Could you check a few things on this drawing? It's one solid part, dimensions in mm from its lowest x, y, z. Give positions to 0.01 mm unless a question says otherwise; leave off trailing zeros. Loops run counter-clockwise (first coordinate to the right, second up) from the corner with the lowest first, then second, coordinate; pieces in that order, holes last. Notation, with made-up numbers: M 85,49 L 134,49 A13 ccw 134,63 Z; hole C 1.5,73.25 d5. An arc over 180 degrees is marked long. Answer as CSV lines item,"result". Start each with the question number.
Item 1: I want a section at B-B on x = 15.25. List the corners of the cut face in (y, z) for me.
Item 2: I want a section at D-D on x = 4. List the corners of the cut face in (y, z) for me, plus the area to 3 significant figures.
Item 3: I want a section at C-C on z = 11.9. List the corners of the cut face in (x, y) for me.
Item 4: If I drill on line 1 along X through (y, z) = (4.55, 42.5); line 2 along Z through (x, y) = (11, 1.25); line 3 along X through (y, z) = (0.45, 11.9), over which ranges is the centre line in solid material (lowest first)? Write a range as from..to.
Item 5: Will these pins go through, and if not, where does the flat tip stop? P1, Ø12, axis at x = 7.5, z = 14, coming from the +Y side; P2, Ø6, axis at x = 15, z = 5, coming from the -Y side; P3, Ø5, axis at x = 18, z = 38.5, coming from the -Y side.
Item 6: If we mould it in two halves opening along Z, with no side actions, what happens to the marked faces 1, 2 and 3? For each: released by +Z, released by -Z, zero draft, split by the parting line, or undercut.
Item 7: I want a section at A-A on y = 3.45. List the corners of the cut face in (x, z) for me.
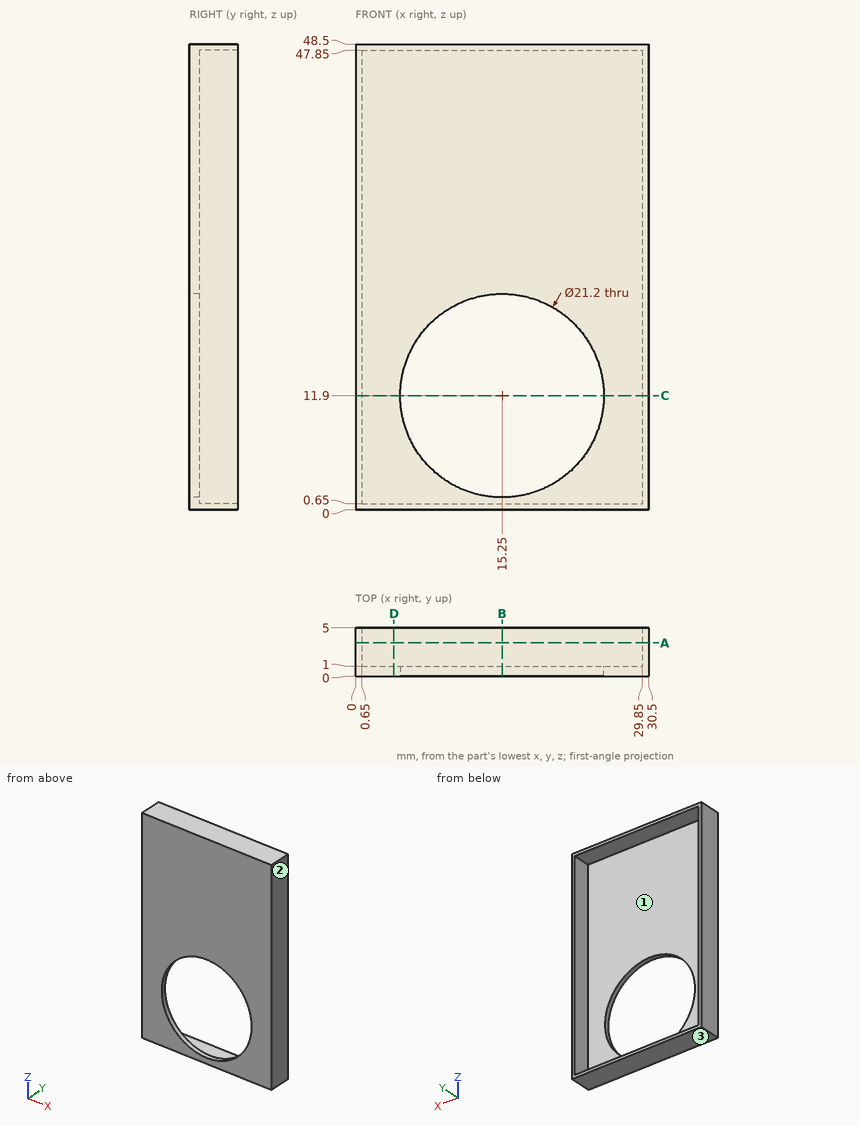
Result:
1,outline,"M 0,0 L 5,0 L 5,0.65 L 1,0.65 L 1,1.3 L 0,1.3 Z; M 0,22.5 L 1,22.5 L 1,47.85 L 5,47.85 L 5,48.5 L 0,48.5 Z"
2,outline,"M 0,0 L 5,0 L 5,0.65 L 1,0.65 L 1,47.85 L 5,47.85 L 5,48.5 L 0,48.5 Z"
2,area,"53.7 mm^2"
3,outline,"M 0,0 L 4.65,0 L 4.65,1 L 0.65,1 L 0.65,5 L 0,5 Z; M 25.85,0 L 30.5,0 L 30.5,5 L 29.85,5 L 29.85,1 L 25.85,1 Z"
4,line 1,"0..0.65, 29.85..30.5"
4,line 2,"0..0.65, 47.85..48.5"
4,line 3,"0..4.65, 25.85..30.5"
5,P1,"y = 1"
5,P2,"through"
5,P3,"y = 0"
6,face 1,"undercut"
6,face 2,"zero draft"
6,face 3,"released by -Z"
7,outline,"M 0,0 L 30.5,0 L 30.5,48.5 L 0,48.5 Z; hole M 0.65,0.65 L 29.85,0.65 L 29.85,47.85 L 0.65,47.85 Z"
